Could you check a few things on this drawing? It's one solid part, dimensions in mm from its lowest x, y, z. Round coordinates to 2 decimals unless told otherwise and drop trailing zeros. Write each loop counter-clockwise with the first axis right and the second up, starting at its lowest first coordinate (ties: lowest second). Pieces come first, ordered by that corner, then holes. Notation, with made-up numbers: M -33,30 L 4,30 A18 ccw 4,63 Z; hole C 61,41.25 d8. An arc over 180 degrees is marked long. One line per item, written item: value. Start each with the question number.
(1) I want a section at A-A on y = 22. Please give me the cut outline in (x, z).
(2) Thinking about a two-plate mould opening in X: for the marked faces 1, 2, 3 and 4, which applies, released by +X, released by -X, zero draft, split by the parting line, or undercut?
(3) If I drill on L1, parallel to X at y = 37.5, z = 3.5 (1 decimal); L2, parallel to X at y = 23.5, z = 6; L3, parallel to Y at x = 18, z = 4.5, over which ranges is the centre line in solid material (lowest first)?
(4) I want a section at D-D on x = 35. Please give me the cut outline in (y, z) (1 decimal), and give its area (3 significant figures).
(5) I'm going to push flat-ended pins straight in: pin 1 Ø3 at (y, z) = (6, 13.5) entering from +X (1 decimal); pin 2 Ø8 at (x, z) = (25, 4.5) entering from +Y; pin 3 Ø5 at (y, z) = (34.5, 16.5) entering from +X. Where does each tip first touch, or does it pass through?
(6) I want a section at B-B on x = 29. Please give me the cut outline in (y, z) (1 decimal), and give its area (3 significant figures).
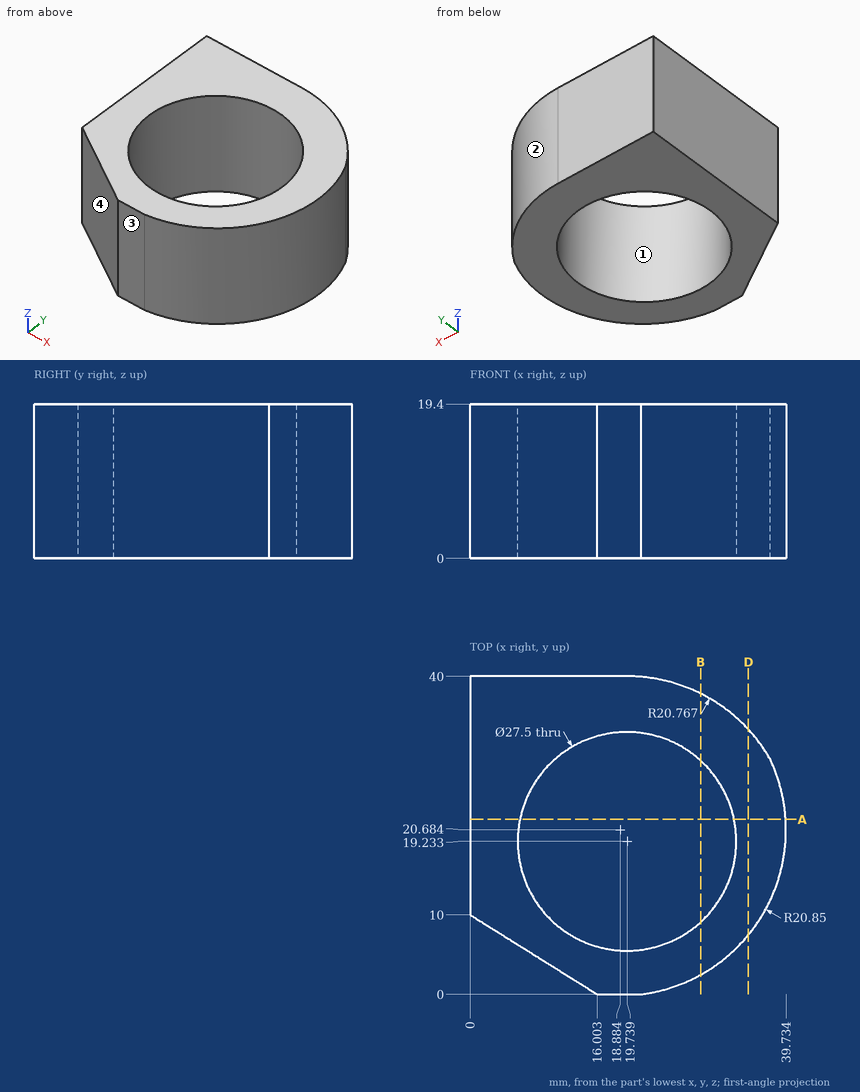
Found:
1. outline: M 0,0 L 6.27,0 L 6.27,19.4 L 0,19.4 Z; M 33.21,0 L 39.69,0 L 39.69,19.4 L 33.21,19.4 Z
2. face 1: undercut
2. face 2: released by +X
2. face 3: zero draft
2. face 4: released by -X
3. L1: x = 0 to 29.6
3. L2: x = 0 to 6.67, 32.81 to 39.54
3. L3: y = 0 to 5.59, 32.87 to 40
4. outline: M 7.5,0 L 33.3,0 L 33.3,19.4 L 7.5,19.4 Z
4. area: 502 mm²
5. pin 1: stops at x = 35
5. pin 2: stops at y = 39.96
5. pin 3: stops at x = 36.12
6. outline: M 2.5,0 L 9.1,0 L 9.1,19.4 L 2.5,19.4 Z; M 29.4,0 L 37.8,0 L 37.8,19.4 L 29.4,19.4 Z
6. area: 292 mm²
